from build123d import *

# Parameters (mm, degrees)
F0_W     = 74.0097276866
F0_H     = 111.5253269672
F1_DEPTH = 19.05
F2_W     = 74.0097276866
F2_H     = 27.8478488326
F3_DEPTH = 114.3
F4_DEPTH = 50.8
F5_W     = 74.0097276866
F5_H     = 13.872501123
F6_DEPTH = 12.7


with BuildPart() as f1:
    # F0 (on Top) → F1 (new body)
    with BuildSketch(Plane.XY):
        with Locations((-5.4957885295, -19.080080092)):
            Rectangle(F0_W, F0_H)
    extrude(amount=F1_DEPTH)

    # F2 (on face) → F3 (join)
    with BuildSketch(Plane.XY.offset(19.05)):
        with Locations((-5.4957885295, -60.9188191593)):
            Rectangle(F2_W, F2_H)
    extrude(amount=F3_DEPTH)

    # F4 (add): a face of the model
    f4_faces = [f1.faces().sort_by_distance(p)[0] for p in [
        (-5.4957885295, 36.6825833917, 9.525),
    ]]
    extrude(f4_faces, amount=F4_DEPTH)

    # F5 (on face) → F6 (join)
    with BuildSketch(Plane.XY.offset(19.05)):
        with Locations((-5.4957885295, 80.5463328302)):
            Rectangle(F5_W, F5_H)
    extrude(amount=F6_DEPTH)


solid = f1.part
Check sheet for the modelled part. Datum: model origin and axes. Units: mm. A direction names the side the tool comes from. Give positions to 0.01 mm unless a question says otherwise; leave off trailing zeros. Loops run counter-clockwise (first coordinate to the right, second up) from the corner with the lowest first, then second, coordinate; pieces in that order, holes last. Notation, with made-up numbers: M 65.5,51 L 102.5,51 A17 cw 102.5,81 Z; hole C 24.25,-6 d11. An arc over 180 degrees is marked long. Return JSON: item names as keys, results as strings. Group by question number.
1. Thickness scan on L1, parallel to Y at x = -14, z = 26; L2, parallel to Y at x = 1, z = 63; L3, parallel to Z at x = -16, y = 25.5. Record the ranges inside material, lowest first.
2. Cross-section at C-C on y = 19.5. Record the boundary of the cut face in (x, z), plus the area to 3 significant figures.
3. Cross-section at B-B on x = -32. Record the boundary of the cut face in (y, z), plus the area to 3 significant figures.
4. Go/stop test with flat-tipped pins: pin 1 (10 mm diameter, centred on y = 47, z = 28, fed in from -X); pin 2 (10 mm diameter, centred on x = 14, y = 20.5, fed in from +Z); pin 3 (11 mm diameter, centred on x = -6, y = 82, fed in from +Z); pin 4 (3 mm diameter, centred on x = -20, z = 113, fed in from +Y). Record where each tip stops, or that it passes through.
5. Cross-section at D-D on y = 77.5. Record the boundary of the cut face in (x, z), plus the area to 3 significant figures.
6. Cross-section at A-A on z = 23.5. Record the boundary of the cut face in (x, y), plus the area to 3 significant figures.
7. Tool access check on faces 5 (the flat face through (-6, 5, 0)), 6 (the flat face through (-6, 73.61, 25)), 7 (the flat face through (-6, 81, 31.75)). Record the directions out of +Z, -Z, +X, -X, +Y, -Y that give a thin tool (end or side, any length) a straight path to the whole face; none if there is none.
8. Mould release check, pull along Y, two halves, no side actions. Record for faces 1 (the flat face through (31.509, -48, 42)), 2 (the flat face through (-6, 87.483, 16)), 3 (the flat face through (-6, 12, 19.05)), 4 (the flat face through (-6, -74.843, 66)): released by +Y, released by -Y, zero draft, split by the parting line, or undercut.
Return value:
{
 "1": {"L1": "-74.84 to -46.99, 73.61 to 87.48", "L2": "-74.84 to -46.99", "L3": "0 to 19.05"},
 "2": {"outline": "M -42.5,0 L 31.51,0 L 31.51,19.05 L -42.5,19.05 Z", "area": "1,410 mm^2"},
 "3": {"outline": "M -74.84,0 L 87.48,0 L 87.48,31.75 L 73.61,31.75 L 73.61,19.05 L -46.99,19.05 L -46.99,133.35 L -74.84,133.35 Z", "area": "6,450 mm^2"},
 "4": {"pin 1": "through", "pin 2": "z = 19.05", "pin 3": "z = 31.75", "pin 4": "y = -46.99"},
 "5": {"outline": "M -42.5,0 L 31.51,0 L 31.51,31.75 L -42.5,31.75 Z", "area": "2,350 mm^2"},
 "6": {"outline": "M -42.5,-74.84 L 31.51,-74.84 L 31.51,-46.99 L -42.5,-46.99 Z; M -42.5,73.61 L 31.51,73.61 L 31.51,87.48 L -42.5,87.48 Z", "area": "3,090 mm^2"},
 "7": {"face 5": "-Z, +X, -X, +Y, -Y", "face 6": "+Z, +X, -X", "face 7": "+Z, +X, -X, +Y"},
 "8": {"face 1": "zero draft", "face 2": "released by +Y", "face 3": "undercut", "face 4": "released by -Y"}
}
